The model under review builds one solid part; all positions refer to its coordinate system, in mm. A direction names the side the tool comes from. Round coordinates to 2 decimals unless told otherwise and drop trailing zeros. Order: outer loops, then holes, each group sorted by start corner. A loop starts at its lowest first (then second) coordinate and runs counter-clockwise, first axis right, second up.
1) Consider section C-C (y = 58). Give the boundary of the cut face in (x, z).
2) Consider section B-B (z = 0). Give the boundary of the cut face in (x, y).
3) Mouldability with a two-part tool opening along Z and no side actions: class faces 4 (the face through (-42, 5, 10)), 5 (the face through (9.76, 145.07, 31)), 6 (the face through (19, 18, -19)), 7 (the face through (-22, 0, 0)) as pulls with the +Z half, pulls with the -Z half, needs draft (parallel to the pull), parting line crosses it, or undercut.
4) Consider section A-A (x = 0). Give the boundary of the cut face in (y, z).
5) Clearance check with flat-ended pins moving along their axes: P1, Ø8, axis at y = 95, z = -3, coming from the -X side; P2, Ø12, axis at x = -9, y = 45.5, coming from the -Z side; P3, Ø10, axis at y = 83.5, z = -7.5, coming from the +X side. State where each tip first meets the part, or that it passes through.
6) Machinability: for faces 1 (the face through (-19, 18, -19)), 2 (the face through (-42, 5, -10)), 3 (the face through (-14.17, 73.95, 34.18)), which of the approach directions +Z, -Z, +X, -X, +Y, -Y give a long, thin tool a straight path to every point of the face, cutting with its end or side? Answer none if there is none.
7) Consider section D-D (z = -29). Give the boundary of the cut face in (x, y), then the cut area to 3 significant figures.
8) To check wall thickness, follow L1, parallel to Z at x = 0, y = 144; L2, parallel to Y at x = 25, z = -18. State the ranges of each line that lie inside material, in increasing order.
from build123d import *

# Parameters (mm, degrees)
SKETCH1_R           = 37
BOSS_EXTRUDE1_DEPTH = 150
SKETCH2_W           = 23
SKETCH2_H           = 23
CUT_EXTRUDE1_DEPTH  = 150
SKETCH3_W           = 43
SKETCH3_H           = 43
CUT_EXTRUDE2_DEPTH  = 36
CHAMFER1_SIZE       = 5
SKETCH5_R           = 32.5
CUT_EXTRUDE3_DEPTH  = 10
SKETCH11_W          = 44.607289856
SKETCH11_H          = 47.277792796
CUT_EXTRUDE7_DEPTH  = 104
SKETCH12_W          = 26
SKETCH12_H          = 20
BOSS_EXTRUDE2_DEPTH = 10
SKETCH13_W          = 20
SKETCH13_H          = 31
CUT_EXTRUDE8_DEPTH  = 11


with BuildPart() as part:
    # Sketch1 → Boss-Extrude1 (new body)
    with BuildSketch(Plane(origin=(0, 0, 0), x_dir=(1, 0, 0), z_dir=(0, 1, 0))):
        with Locations(Location((0, 0, 0), (0, 0, 270))):
            Circle(SKETCH1_R)
    extrude(amount=BOSS_EXTRUDE1_DEPTH)

    # Sketch2 → Cut-Extrude1 (cut)
    with BuildSketch(Plane(origin=(0, 150, 0), x_dir=(1, 0, 0), z_dir=(0, 1, 0))):
        Rectangle(SKETCH2_W, SKETCH2_H)
    extrude(amount=-CUT_EXTRUDE1_DEPTH, mode=Mode.SUBTRACT)

    # Sketch3 → Cut-Extrude2 (cut)
    with BuildSketch(Plane.XZ):
        Rectangle(SKETCH3_W, SKETCH3_H)
    extrude(amount=-CUT_EXTRUDE2_DEPTH, mode=Mode.SUBTRACT)

    # Chamfer1
    chamfer1_edges = [part.edges().sort_by_distance(p)[0] for p in [
        (21.5, 18, 21.5),
        (21.5, 18, -21.5),
        (-21.5, 18, -21.5),
        (-21.5, 18, 21.5),
    ]]
    chamfer(chamfer1_edges, length=CHAMFER1_SIZE)

    # Sketch5 → Cut-Extrude3 (cut)
    with BuildSketch(Plane(origin=(0, 150, 0), x_dir=(1, 0, 0), z_dir=(0, 1, 0))):
        with Locations(Location((0, 0, 0), (0, 0, 270))):
            Circle(SKETCH5_R)
    extrude(amount=-CUT_EXTRUDE3_DEPTH, mode=Mode.SUBTRACT)

    # Sketch11 → Cut-Extrude7 (cut)
    with BuildSketch(Plane(origin=(0, 140, 0), x_dir=(1, 0, 0), z_dir=(0, 1, 0))):
        Rectangle(SKETCH11_W, SKETCH11_H)
    extrude(amount=-CUT_EXTRUDE7_DEPTH, mode=Mode.SUBTRACT)

    # Sketch12 → Boss-Extrude2 (add)
    with BuildSketch(Plane.XZ):
        with Locations((-34.5, 0)):
            Rectangle(SKETCH12_W, SKETCH12_H)
        with Locations((34.5, 0)):
            Rectangle(SKETCH12_W, SKETCH12_H)
    extrude(amount=-BOSS_EXTRUDE2_DEPTH)

    # Sketch13 → Cut-Extrude8 (cut)
    with BuildSketch(Plane.XZ):
        with Locations((0, 37)):
            Rectangle(SKETCH13_W, SKETCH13_H)
    extrude(amount=-CUT_EXTRUDE8_DEPTH, mode=Mode.SUBTRACT)


solid = part.part
Answer below:
1. outline: circle Ø74 at (0, 0); hole (-22.3, -23.64) - (22.3, -23.64) - (22.3, 23.64) - (-22.3, 23.64) - close
2. outline: (-47.5, 0) - (-21.5, 0) - (-21.5, 36) - (-22.3, 36) - (-22.3, 140) - (-32.5, 140) - (-32.5, 150) - (-37, 150) - (-37, 10) - (-47.5, 10) - close; (21.5, 0) - (47.5, 0) - (47.5, 10) - (37, 10) - (37, 150) - (32.5, 150) - (32.5, 140) - (22.3, 140) - (22.3, 36) - (21.5, 36) - close
3. face 4: pulls with the +Z half
3. face 5: undercut
3. face 6: undercut
3. face 7: needs draft
4. outline: (0, -37) - (150, -37) - (150, -32.5) - (140, -32.5) - (140, -23.64) - (36, -23.64) - (36, -21.5) - (0, -21.5) - close; (11, 21.5) - (36, 21.5) - (36, 23.64) - (140, 23.64) - (140, 32.5) - (150, 32.5) - (150, 37) - (11, 37) - close
5. P1: stops at x = -37
5. P2: stops at z = -36.88
5. P3: stops at x = 36.92
6. face 1: +Y, -Y
6. face 2: -Z, -X, +Y, -Y
6. face 3: +Y
7. outline: (-22.98, 0) - (22.98, 0) - (22.98, 150) - (14.67, 150) - (14.67, 140) - (-14.67, 140) - (-14.67, 150) - (-22.98, 150) - close
7. area: 6,600 mm2
8. L1: z = -37 to -32.5, 32.5 to 37
8. L2: y = 0 to 140
